from build123d import *

# Parameters (mm, degrees)
F0_W     = 50
F0_H     = 65
F1_DEPTH = 13.8
F2_R     = 109
F3_DEPTH = 65
F5_DEPTH = 15


with BuildPart() as f1:
    # F0 (on Top) → F1 (new body)
    with BuildSketch(Plane.XY):
        Rectangle(F0_W, F0_H)
    extrude(amount=F1_DEPTH)

    # F2 (on face) → F3 (cut)
    with BuildSketch(Plane(origin=(0, 32.5, 0), x_dir=(-1, 0, 0), z_dir=(0, 1, 0))):
        with Locations((0, 119.894297679)):
            Circle(F2_R)
    extrude(amount=-F3_DEPTH, mode=Mode.SUBTRACT)

    # F4 (on face) → F5 (cut)
    with BuildSketch(Plane(origin=(0, 0, 0), x_dir=(1, 0, 0), z_dir=(0, 0, -1))):
        with BuildLine():
            ThreePointArc((-17, 21.5), (-15, 19.5), (-13, 21.5))
            Line((-13, 21.5), (-17, 21.5))
        make_face()
        with BuildLine():
            Line((-17, 21.5), (-13, 21.5))
            ThreePointArc((-13, 21.5), (-15, 23.5), (-17, 21.5))
        make_face()
        with BuildLine():
            Line((-13, -8.5), (-13, 21.5))
            ThreePointArc((-13, 21.5), (-15, 19.5), (-17, 21.5))
            Line((-17, 21.5), (-17, -8.5))
            ThreePointArc((-17, -8.5), (-15, -6.5), (-13, -8.5))
        make_face()
        with BuildLine():
            ThreePointArc((-17, -8.5), (-15, -10.5), (-13, -8.5))
            Line((-13, -8.5), (-17, -8.5))
        make_face()
        with BuildLine():
            Line((-17, -8.5), (-13, -8.5))
            ThreePointArc((-13, -8.5), (-15, -6.5), (-17, -8.5))
        make_face()
        with BuildLine():
            ThreePointArc((17, 21.5), (15, 23.5), (13, 21.5))
            Line((13, 21.5), (17, 21.5))
        make_face()
        with BuildLine():
            ThreePointArc((17, 21.5), (15, 19.5), (13, 21.5))
            Line((13, 21.5), (13, -8.5))
            ThreePointArc((13, -8.5), (15, -6.5), (17, -8.5))
            Line((17, -8.5), (17, 21.5))
        make_face()
        with BuildLine():
            Line((17, 21.5), (13, 21.5))
            ThreePointArc((13, 21.5), (15, 19.5), (17, 21.5))
        make_face()
        with BuildLine():
            ThreePointArc((17, -8.5), (15, -6.5), (13, -8.5))
            Line((13, -8.5), (17, -8.5))
        make_face()
        with BuildLine():
            Line((17, -8.5), (13, -8.5))
            ThreePointArc((13, -8.5), (15, -10.5), (17, -8.5))
        make_face()
    extrude(amount=-F5_DEPTH, mode=Mode.SUBTRACT)


solid = f1.part
The listing builds one solid part. Answer for the finished solid, in the listing's coordinates (mm). A direction names the side the tool comes from. Give positions to 0.01 mm unless a question says otherwise; leave off trailing zeros. Write each loop counter-clockwise with the first axis right and the second up, starting at its lowest first coordinate (ties: lowest second). Pieces come first, ordered by that corner, then holes.
1) Section D-D (y = 25) is taken. Write down the section's boundary in (x, z), and give its area (3 significant figures).
2) Given P1, Ø5, axis at x = -9, y = 21, coming from the +Z side, flat-ended and moving along its own axis, determine where the tip first touches the part or whether it passes through.
3) Section C-C (x = 15) is taken. Write down the section's boundary in (y, z), and give its area (3 significant figures).
4) Section B-B (z = 5) is taken. Write down the section's boundary in (x, y).
5) Find the intervals of material crossed by L1, parallel to X at y = -16, z = 4.5; L2, parallel to X at y = -18, z = 11.75; L3, parallel to Y at x = -15, z = 10.75, in increasing order.
6) For a pull along X with two mould halves and no side action, classify faces 1 (the face through (25, 0, 7)), 2 (the face through (0, 0, 0)), 3 (the face through (-17, -7, 6)), 4 (the face through (15, -23.5, 6)) as pulls with the +X half, pulls with the -X half, needs draft (parallel to the pull), parting line crosses it, or undercut.
7) Section A-A (y = -9) is taken. Write down the section's boundary in (x, z), and give its area (3 significant figures).
8) A tool of negligible diameter and unlimited length cuts with its end or side. For faces 5 (the face through (-13, -6, 6)), 6 (the face through (0, 32.5, 5)), from which of +Z, -Z, +X, -X, +Y, -Y can it reach the whole face along a straight path? Write none if from no direction.
Response:
1. outline: (-25, 0) - (25, 0) - (25, 13.8) arc R109 cw to (-25, 13.8) - close
1. area: 593 mm2
2. P1: stops at z = 11.5
3. outline: (-32.5, 0) - (-23.5, 0) - (-23.5, 11.93) - (-32.5, 11.93) - close; (10.5, 0) - (32.5, 0) - (32.5, 11.93) - (10.5, 11.93) - close
3. area: 370 mm2
4. outline: (-25, -32.5) - (25, -32.5) - (25, 32.5) - (-25, 32.5) - close; hole (-17, -21.5) arc R2 ccw to (-13, -21.5) - (-13, 8.5) arc R2 ccw to (-17, 8.5) - close; hole (13, -21.5) arc R2 ccw to (17, -21.5) - (17, 8.5) arc R2 ccw to (13, 8.5) - close
5. L1: x = -25 to -17, -13 to 13, 17 to 25
5. L2: x = -25 to -17, 17 to 25
5. L3: y = -32.5 to -23.5, 10.5 to 32.5
6. face 1: pulls with the +X half
6. face 2: needs draft
6. face 3: undercut
6. face 4: undercut
7. outline: (-25, 0) - (-17, 0) - (-17, 12.23) arc R109 cw to (-25, 13.8) - close; (-13, 0) - (13, 0) - (13, 11.67) arc R109 cw to (-13, 11.67) - close; (17, 0) - (25, 0) - (25, 13.8) arc R109 cw to (17, 12.23) - close
7. area: 497 mm2
8. face 5: +Z, -Z
8. face 6: +Z, -Z, +X, -X, +Y
